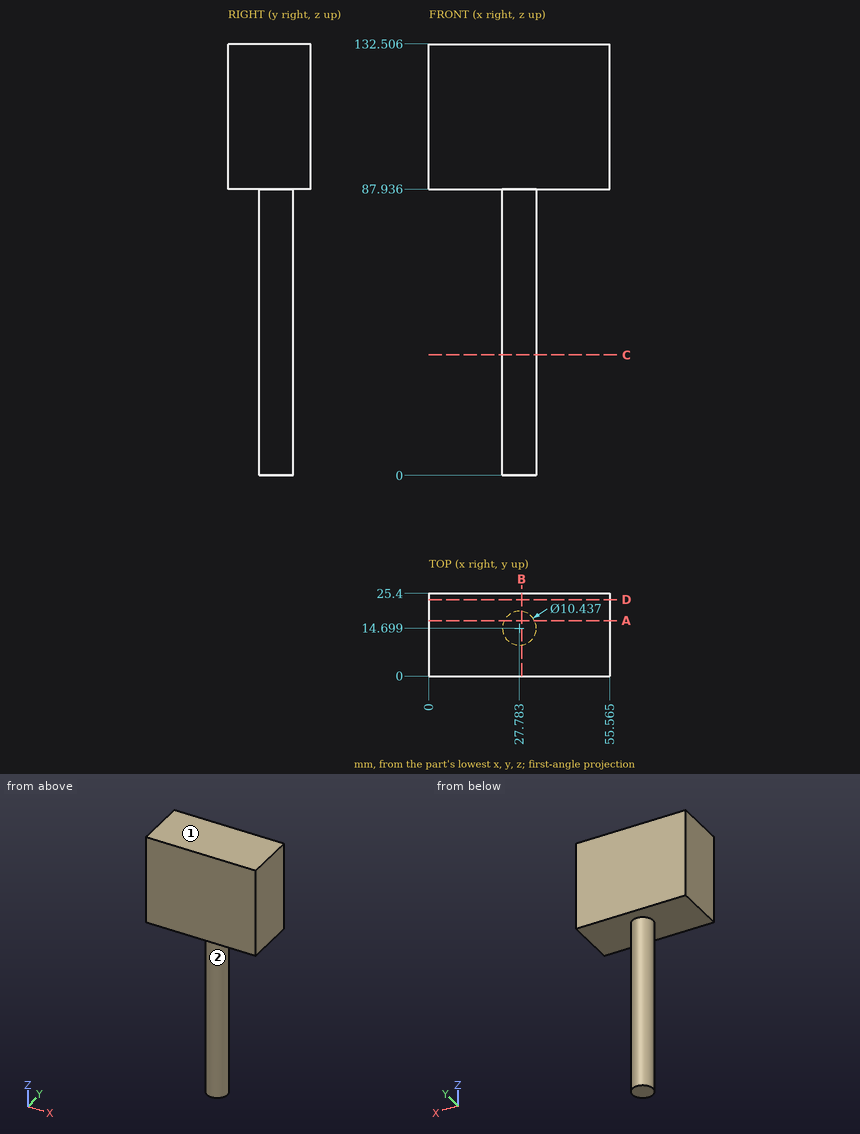
Geometry check sheet. Reference: drawing and pictorial views, mm from the part's lowest x, y, z. A direction names the side the tool comes from. Round coordinates to 2 decimals unless told otherwise and drop trailing zeros. Loops run counter-clockwise (first coordinate to the right, second up) from the corner with the lowest first, then second, coordinate; pieces in that order, holes last. Notation, with made-up numbers: (83, -15) - (98, -15) arc R30 cw to (98, 14) - close; hole circle Ø10 at (66.5, 14). An arc over 180 degrees is marked (long way). Answer in a Markdown table with one row per item. Add a question column.
Q1. Section check D-D on y = 23.5. Enter the section's corners in (x, z) (1 decimal), plus the area to 3 significant figures.
Q2. Gauge pin test, flat ends, axial feed: pin 1 (6 mm diameter, centred on y = 9.5, z = 71, fed in from -X); pin 2 (5 mm diameter, centred on y = 8, z = 40.5, fed in from -X) (1 decimal). Record the tip position at first contact, or that the pin passes through.
Q3. Material ranges on line 1 (Z direction, x = 9.5, y = 21.25) (1 decimal); line 2 (X direction, y = 15, z = 36.5); line 3 (X direction, y = 10.5, z = 62) (1 decimal), recorded low to high.
Q4. Tool access check on the marked faces 1 and 2. Record the directions out of +Z, -Z, +X, -X, +Y, -Y that give a thin tool (end or side, any length) a straight path to the whole face; none if there is none.
Q5. Section check A-A on y = 17. Enter the section's corners in (x, z) (1 decimal), plus the area to 3 significant figures.
Q6. Section check C-C on z = 37. Enter the section's corners in (x, y).
Q7. Section check B-B on x = 28.5. Enter the section's corners in (y, z) (1 decimal).
Found:
| question | item | result |
|---|---|---|
| 1 | outline | (0, 87.9) - (55.6, 87.9) - (55.6, 132.5) - (0, 132.5) - close |
| 1 | area | 2,480 mm² |
| 2 | pin 1 | stops at x = 23.05 |
| 2 | pin 2 | stops at x = 24.7 |
| 3 | line 1 | z = 87.9 to 132.5 |
| 3 | line 2 | x = 22.57 to 32.99 |
| 3 | line 3 | x = 24.7 to 30.9 |
| 4 | face 1 | +Z, +X, -X, +Y, -Y |
| 4 | face 2 | -Z |
| 5 | outline | (0, 87.9) - (23.1, 87.9) - (23.1, 0) - (32.5, 0) - (32.5, 87.9) - (55.6, 87.9) - (55.6, 132.5) - (0, 132.5) - close |
| 5 | area | 3,300 mm² |
| 6 | outline | circle Ø10.44 at (27.78, 14.7) |
| 7 | outline | (0, 87.9) - (9.5, 87.9) - (9.5, 0) - (19.9, 0) - (19.9, 87.9) - (25.4, 87.9) - (25.4, 132.5) - (0, 132.5) - close |
